```python
from build123d import *

# Parameters (mm, degrees)
SKETCH1_R           = 6
BOSS_EXTRUDE1_DEPTH = 4
SKETCH2_R           = 2.4
CUT_EXTRUDE1_DEPTH  = 9
SKETCH3_R           = 11
SKETCH3_R_2         = 6
BOSS_EXTRUDE2_DEPTH = 27


with BuildPart() as part:
    # Sketch1 → Boss-Extrude1 (new body, symmetric)
    with BuildSketch(Plane.XY):
        with BuildLine():
            Line((-18.375, 10.166581284), (-18.375, -10.166581284))
            ThreePointArc((-18.375, -10.166581284), (0, -21), (18.375, -10.166581284))
            Line((18.375, -10.166581284), (18.375, 10.166581284))
            ThreePointArc((18.375, 10.166581284), (0, 21), (-18.375, 10.166581284))
        make_face()
        Circle(SKETCH1_R, mode=Mode.SUBTRACT)
    extrude(amount=BOSS_EXTRUDE1_DEPTH, both=True)

    # Sketch2 → Cut-Extrude1 (cut, through all)
    with BuildSketch(Plane.XY.offset(4)):
        with Locations((-11.490485194, 11.490485194)):
            Circle(SKETCH2_R)
        with Locations((0, 16.25)):
            Circle(SKETCH2_R)
        with Locations((11.490485194, 11.490485194)):
            Circle(SKETCH2_R)
        with Locations((11.490485194, -11.490485194)):
            Circle(SKETCH2_R)
        with Locations((0, -16.25)):
            Circle(SKETCH2_R)
        with Locations((-11.490485194, -11.490485194)):
            Circle(SKETCH2_R)
    extrude(amount=-CUT_EXTRUDE1_DEPTH, mode=Mode.SUBTRACT)

    # Sketch3 → Boss-Extrude2 (add)
    with BuildSketch(Plane(origin=(0, 0, -4), x_dir=(-1, 0, 0), z_dir=(0, 0, -1))):
        Circle(SKETCH3_R)
        Circle(SKETCH3_R_2, mode=Mode.SUBTRACT)
    extrude(amount=BOSS_EXTRUDE2_DEPTH)


solid = part.part
```
Can you work these out from the model? Positions are in its coordinate system, mm. A direction names the side the tool comes from. Coordinates: 2 decimals unless noted, no trailing zeros. Write each loop counter-clockwise with the first axis right and the second up, starting at its lowest first coordinate (ties: lowest second). Pieces come first, ordered by that corner, then holes. Notation, with made-up numbers: M -36,0.25 L -27,0.25 A23 cw -27,36.25 Z; hole C -9.75,63.5 d1. An arc over 180 degrees is marked long. Write item = value, one per line. Start each with the question number.
Q1. If we section it at B-B, the plane x = 4.5: Write out the boundary of the cut face in (y, z), then the cut area to 3 significant figures.
Q2. Thinking about a two-plate mould opening in Y: for faces 3 (the face through (0, 21, 0)), 4 (the face through (18.375, 0, 0)), 5 (the face through (1.29, 18.274, 0.056)), which applies, released by +Y, released by -Y, zero draft, split by the parting line, or undercut?
Q3. On a 3-axis mill with a long thin cutter (end or side, diameter ignored), from which of +Z, -Z, +X, -X, +Y, -Y can I reach the whole of each face in a straight line? I mean faces 1 (the face through (2.38, -10.74, -17.31)), 2 (the face through (13.707, -12.41, 0.056)). Say none if no direction works.
Q4. If I drill on L1, parallel to Z at x = -13.5, y = 6; L2, parallel to Y at x = -3, z = -15.5; L3, parallel to Y at x = -12.5, z = 2, over which ranges is the centre line in solid material (lowest first)? Write a range as [from, to].
Q5. If we section it at D-D, the plane z = -3: Write out the boundary of the cut face in (x, y) (3 decimals).
Q6. If we section it at C-C, the plane y = -16.25: Write out the boundary of the cut face in (x, z), then the cut area to 3 significant figures.
Q7. If we section it at A-A, the plane x = 0: Write out the boundary of the cut face in (y, z), then the cut area to 3 significant figures.
Q8. I'm going to push flat-ended pins straight in: pin 1 (1 mm diameter, centred on x = 12, y = -15, fed in from -Z); pin 2 (6 mm diameter, centred on y = 6, z = -14.5, fed in from +X); pin 3 (8 mm diameter, centred on y = 9, z = -15, fed in from +X); pin 4 (1 mm diameter, centred on x = -12, z = -13.5, fed in from +Y). Where does each tip first touch, or does it pass through?
Check sheet entries:
q1.outline = M -20.51,-4 L -10.04,-4 L -10.04,-31 L -3.97,-31 L -3.97,4 L -20.51,4 Z; M 3.97,-31 L 10.04,-31 L 10.04,-4 L 20.51,-4 L 20.51,4 L 3.97,4 Z
q1.area = 592 mm²
q2.face_3 = released by +Y
q2.face_4 = zero draft
q2.face_5 = undercut
q3.face_1 = -Z
q3.face_2 = +Z, -Z
q4.L1 = [-4, 4]
q4.L2 = [-10.58, -5.2], [5.2, 10.58]
q4.L3 = [-16.87, -13.67], [-9.31, 9.31], [13.67, 16.87]
q5.outline = M -18.375,-10.167 A21 ccw 18.375,-10.167 L 18.375,10.167 A21 ccw -18.375,10.167 Z; hole C -11.49,-11.49 d4.8; hole C -11.49,11.49 d4.8; hole C 0,0 d12; hole C 0,-16.25 d4.8; hole C 0,16.25 d4.8; hole C 11.49,-11.49 d4.8; hole C 11.49,11.49 d4.8
q6.outline = M -13.3,-4 L -2.4,-4 L -2.4,4 L -13.3,4 Z; M 2.4,-4 L 13.3,-4 L 13.3,4 L 2.4,4 Z
q6.area = 174 mm²
q7.outline = M -21,-4 L -18.65,-4 L -18.65,4 L -21,4 Z; M -13.85,-4 L -11,-4 L -11,-31 L -6,-31 L -6,4 L -13.85,4 Z; M 6,-31 L 11,-31 L 11,-4 L 13.85,-4 L 13.85,4 L 6,4 Z; M 18.65,-4 L 21,-4 L 21,4 L 18.65,4 Z
q7.area = 433 mm²
q8.pin_1 = -4
q8.pin_2 = 10.58
q8.pin_3 = 9.8
q8.pin_4 = through
